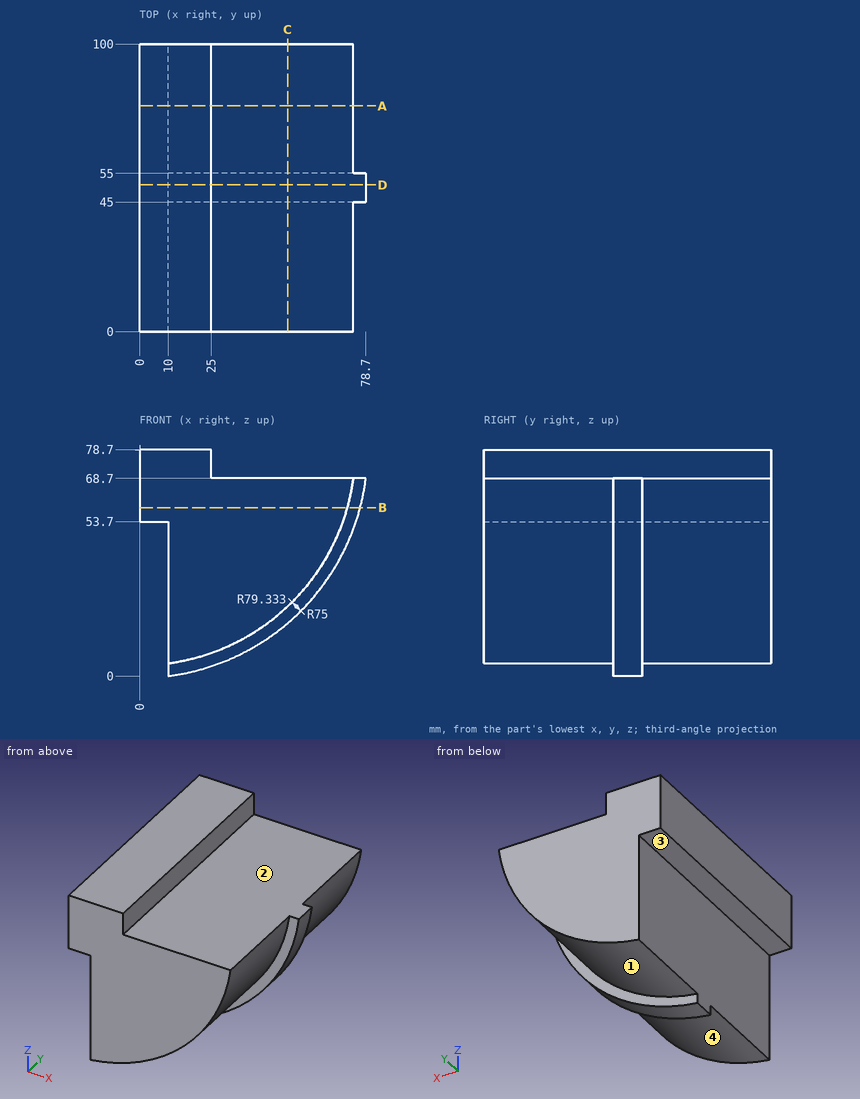
The figure shows three views and two pictorial views of one solid part (mm, origin at its lowest corner). Answer the questions. A direction names the side the tool comes from. Give positions to 0.01 mm unless a question says otherwise; leave off trailing zeros. Write each loop counter-clockwise with the first axis right and the second up, starting at its lowest first coordinate (ties: lowest second). Pieces come first, ordered by that corner, then holes. Notation, with made-up numbers: (-16, 18) -> (36, 18) arc R25 cw to (36, 37) -> close; hole circle Ø3 at (-31, -1). An arc over 180 degrees is marked (long way). Write each question's results on one line, items separated by ' | '.
1. Each of these flat-tipped pins is pushed along its axis until it touches: pin 1 Ø12 at (y, z) = (16, 24.5) entering from -X; pin 2 Ø1 at (x, y) = (65, 35.5) entering from +Z; pin 3 Ø6 at (x, z) = (55.5, 27.5) entering from -Y; pin 4 Ø3 at (x, y) = (7, 35.5) entering from -Z. Where does it stop, or does it pass through?
Data:
pin 1: x = 10 | pin 2: z = 68.7 | pin 3: y = 0 | pin 4: z = 53.7
2. Find section C-C on x = 51.5. Determine the outline of the cut face in (y, z), and give its area (3 significant figures).
Data:
outline: (0, 24.18) -> (45, 24.18) -> (45, 18.36) -> (55, 18.36) -> (55, 24.18) -> (100, 24.18) -> (100, 68.7) -> (0, 68.7) -> close | area: 4,510 mm^2
3. Straight lines are drawn through the part: L1, parallel to Z at x = 5.5, y = 50.5; L2, parallel to X at y = 22.5, z = 71.5; L3, parallel to Y at x = 36, z = 12.5. For each, find the intervals that lie inside material, in ascending order.
Data:
L1: 53.7 to 78.7 | L2: 0 to 25 | L3: 45 to 55
4. Find section D-D on y = 51. Determine the outline of the cut face in (x, z), and give its area (3 significant figures).
Data:
outline: (0, 53.7) -> (10, 53.7) -> (10, 0) arc R79.33 ccw to (78.7, 68.7) -> (25, 68.7) -> (25, 78.7) -> (0, 78.7) -> close | area: 3,860 mm^2
5. A tool of negligible diameter and unlimited length cuts with its end or side. For the marked faces 1, 2, 3 and 4, from which of +Z, -Z, +X, -X, +Y, -Y can it reach the whole face along a straight path? Write none if from no direction.
Data:
face 1: -Z, +X, +Y | face 2: +Z, +X, +Y, -Y | face 3: -Z, -X, +Y, -Y | face 4: -Z, +X, -Y
6. Find section B-B on z = 58.5. Determine the outline of the cut face in (x, y).
Data:
outline: (0, 0) -> (72.23, 0) -> (72.23, 45) -> (76.72, 45) -> (76.72, 55) -> (72.23, 55) -> (72.23, 100) -> (0, 100) -> close
7. Find section A-A on y = 78.5. Determine the outline of the cut face in (x, z), and give its area (3 significant figures).
Data:
outline: (0, 53.7) -> (10, 53.7) -> (10, 4.37) arc R75 ccw to (74.33, 68.7) -> (25, 68.7) -> (25, 78.7) -> (0, 78.7) -> close | area: 3,420 mm^2
